```python
from build123d import *

# Parameters (mm, degrees)
SKETCH1_R           = 3.175
SKETCH1_R_2         = 3.2639
SKETCH1_R_3         = 3.96875
SKETCH1_R_4         = 2.38125
BOSS_EXTRUDE1_DEPTH = 3.175


with BuildPart() as part:
    # Sketch1 → Boss-Extrude1 (new body)
    # profile 1 of 7: a face of its own
    with BuildSketch(Plane.ZY.offset(25.4)):
        with BuildLine():
            Line((-88.4975, 379.360683619), (-113.503995941, 354.868900976))
            ThreePointArc((-113.503995941, 354.868900976), (-115.701762144, 347.491113055), (-110.608164688, 341.71900808))
            Line((-110.608164688, 341.71900808), (-88.4975, 333.860683619))
            Line((-88.4975, 333.860683619), (-102.195874596, 351.845168269))
            ThreePointArc((-102.195874596, 351.845168269), (-103.980307482, 357.263971701), (-102.037425504, 362.628003857))
            Line((-102.037425504, 362.628003857), (-88.4975, 379.360683619))
        make_face()
        with Locations((-107.95, 349.198183619)):
            Circle(SKETCH1_R, mode=Mode.SUBTRACT)
    # profile 2 of 7: a face of its own
    with BuildSketch(Plane.ZY.offset(25.4)):
        with BuildLine():
            Line((-54.275, 333.860683619), (-54.275, 379.360683619))
            Line((-54.275, 379.360683619), (-88.4975, 379.360683619))
            Line((-88.4975, 379.360683619), (-102.037425504, 362.628003857))
            ThreePointArc((-102.037425504, 362.628003857), (-103.980307482, 357.263971701), (-102.195874596, 351.845168269))
            Line((-102.195874596, 351.845168269), (-88.4975, 333.860683619))
            Line((-88.4975, 333.860683619), (-54.275, 333.860683619))
        make_face()
        with Locations((-83.735, 340.735683619)):
            Circle(SKETCH1_R_2, mode=Mode.SUBTRACT)
        with Locations((-95.25, 357.135683619)):
            Circle(SKETCH1_R_3, mode=Mode.SUBTRACT)
        with Locations((-60.625, 366.135683619)):
            Circle(SKETCH1_R_2, mode=Mode.SUBTRACT)
        with Locations((-83.735, 372.485683619)):
            Circle(SKETCH1_R_2, mode=Mode.SUBTRACT)
        with Locations((-60.625, 347.085683619)):
            Circle(SKETCH1_R_2, mode=Mode.SUBTRACT)
    # profile 3 of 7: a face of its own
    with BuildSketch(Plane.ZY.offset(25.4)):
        with Locations((-95.25, 357.135683619)):
            Circle(SKETCH1_R_3)
    # profile 4 of 7: a face of its own
    with BuildSketch(Plane.ZY.offset(25.4)):
        with Locations((-60.625, 366.135683619)):
            Circle(SKETCH1_R_2)
        with Locations((-60.625, 366.135683619)):
            Circle(SKETCH1_R_4, mode=Mode.SUBTRACT)
    # profile 5 of 7: a face of its own
    with BuildSketch(Plane.ZY.offset(25.4)):
        with Locations((-83.735, 372.485683619)):
            Circle(SKETCH1_R_2)
        with Locations((-83.735, 372.485683619)):
            Circle(SKETCH1_R_4, mode=Mode.SUBTRACT)
    # profile 6 of 7: a face of its own
    with BuildSketch(Plane.ZY.offset(25.4)):
        with Locations((-60.625, 347.085683619)):
            Circle(SKETCH1_R_2)
        with Locations((-60.625, 347.085683619)):
            Circle(SKETCH1_R_4, mode=Mode.SUBTRACT)
    # profile 7 of 7: a face of its own
    with BuildSketch(Plane.ZY.offset(25.4)):
        with Locations((-83.735, 340.735683619)):
            Circle(SKETCH1_R_2)
        with Locations((-83.735, 340.735683619)):
            Circle(SKETCH1_R_4, mode=Mode.SUBTRACT)
    extrude(amount=BOSS_EXTRUDE1_DEPTH)


solid = part.part
```
Geometry check sheet. Reference: the model listing, model coordinates, mm. Coordinates: 2 decimals unless noted, no trailing zeros. Order: outer loops, then holes, each group sorted by start corner. A loop starts at its lowest first (then second) coordinate and runs counter-clockwise, first axis right, second up.
Item 1: Section check C-C (x = -27.6). Count the separate pieces of the cut face and the enclosed holes in it, plus the area to 3 significant figures.
Item 2: Depth check by flat-ended pin: pin 1 (4 mm diameter, centred on y = 372.49, z = -83.74, fed in from -X). Enter the tip coordinate at first touch or a pass-through.
Item 3: Mould release check, pull along Z, two halves, no side actions. Record for faces 1 (the cylindrical face through (-26.97, 344.76, -61.14)), 2 (the flat face through (-27, 379.361, -71)), 3 (the cylindrical face through (-26.965, 347.601, -115.725)), 4 (the cylindrical face through (-26.97, 363.81, -61.14)): released by +Z, released by -Z, zero draft, split by the parting line, or undercut.
Item 4: Section check B-B (z = -84.5). Enter the section's corners in (x, y) (3 decimals).
Item 5: Scan lines: line 1 along Z through (x, y) = (-27.9, 346.5) (3 decimals); line 2 along Y through (x, z) = (-27.7, -61); line 3 along Z through (x, y) = (-27.35, 364) (3 decimals). Record each from-to range of solid material in increasing order.
Item 6: Section check D-D (z = -107.95). Enter the section's corners in (x, y) (3 decimals).
Item 7: Section check A-A (y = 365.5). Enter the section's corners in (x, z) (3 decimals), plus the area to 3 significant figures.
Check sheet entries:
1. separate pieces: 1
1. enclosed holes: 5
1. area: 2,190 mm2
2. pin 1: passes through
3. face 1: undercut
3. face 2: zero draft
3. face 3: released by -Z
3. face 4: undercut
4. outline: (-28.575, 333.861) - (-25.4, 333.861) - (-25.4, 338.481) - (-28.575, 338.481) - close; (-28.575, 342.991) - (-25.4, 342.991) - (-25.4, 370.231) - (-28.575, 370.231) - close; (-28.575, 374.741) - (-25.4, 374.741) - (-25.4, 379.361) - (-28.575, 379.361) - close
5. line 1: z = -115.415 to -109.623, -106.277 to -62.933, -58.317 to -54.275
5. line 2: y = 333.86 to 344.73, 349.44 to 363.78, 368.49 to 379.36
5. line 3: z = -104.181 to -61.678, -59.572 to -54.275
6. outline: (-28.575, 340.774) - (-25.4, 340.774) - (-25.4, 346.023) - (-28.575, 346.023) - close; (-28.575, 352.373) - (-25.4, 352.373) - (-25.4, 360.309) - (-28.575, 360.309) - close
7. outline: (-28.575, -102.649) - (-25.4, -102.649) - (-25.4, -62.92) - (-28.575, -62.92) - close; (-28.575, -58.33) - (-25.4, -58.33) - (-25.4, -54.275) - (-28.575, -54.275) - close
7. area: 139 mm2
